Geometry: final body of the model. Coordinates: model frame, mm. Coordinates: 2 decimals unless noted, no trailing zeros. Use a Markdown table: item, result. Add a question column.
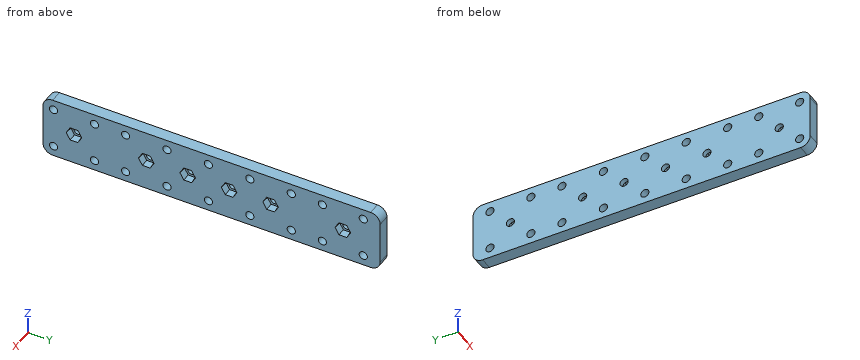
```python
from build123d import *

# Parameters (mm, degrees)
ESQUISSE2_R             = 1.7
BOSS_EXTRU_1_DEPTH      = 5
ENL_V_MAT_EXTRU_1_DEPTH = 3
ENL_V_MAT_EXTRU_1_TAPER = 5


with BuildPart() as part:
    # Esquisse2 → Boss.-Extru.1 (new body)
    with BuildSketch(Plane(origin=(0, 0, 0), x_dir=(0, 0, -1), z_dir=(1, 0, 0))):
        with BuildLine():
            Line((-25.6, -133.893899255), (-25.6, -1.893899255))
            ThreePointArc((-25.6, -1.893899255), (-24.428427125, 0.93452787), (-21.6, 2.106100745))
            Line((-21.6, 2.106100745), (-4.004577751, 2.106100745))
            ThreePointArc((-4.004577751, 2.106100745), (-1.176198229, 0.934575472), (-0.004577753, -1.893764615))
            Line((-0.004577753, -1.893764615), (-0.000134644, -133.893764615))
            ThreePointArc((-0.000134644, -133.893764615), (-1.171659915, -136.722278777), (-4.000134642, -137.893899255))
            Line((-4.000134642, -137.893899255), (-21.6, -137.893899255))
            ThreePointArc((-21.6, -137.893899255), (-24.428427125, -136.72232638), (-25.6, -133.893899255))
        make_face()
        with Locations((-21.285281374, -103.629375049)):
            Circle(ESQUISSE2_R, mode=Mode.SUBTRACT)
        with Locations((-4.314718626, -103.629375049)):
            Circle(ESQUISSE2_R, mode=Mode.SUBTRACT)
        with Locations((-4.314718626, -86.427328272)):
            Circle(ESQUISSE2_R, mode=Mode.SUBTRACT)
        with Locations((-21.285281374, -86.427328272)):
            Circle(ESQUISSE2_R, mode=Mode.SUBTRACT)
        with Locations((-21.285281374, -133.513633034)):
            Circle(ESQUISSE2_R, mode=Mode.SUBTRACT)
        with Locations((-4.314718626, -133.513633034)):
            Circle(ESQUISSE2_R, mode=Mode.SUBTRACT)
        with Locations((-4.314718626, -69.225281495)):
            Circle(ESQUISSE2_R, mode=Mode.SUBTRACT)
        with Locations((-21.285281374, -69.225281495)):
            Circle(ESQUISSE2_R, mode=Mode.SUBTRACT)
        with Locations((-4.314718626, -52.023234718)):
            Circle(ESQUISSE2_R, mode=Mode.SUBTRACT)
        with Locations((-21.285281374, -52.023234718)):
            Circle(ESQUISSE2_R, mode=Mode.SUBTRACT)
        with Locations((-4.314718626, -34.821187941)):
            Circle(ESQUISSE2_R, mode=Mode.SUBTRACT)
        with Locations((-21.285281374, -34.821187941)):
            Circle(ESQUISSE2_R, mode=Mode.SUBTRACT)
        with Locations((-21.285281374, -4.936929955)):
            Circle(ESQUISSE2_R, mode=Mode.SUBTRACT)
        with Locations((-4.314718626, -4.936929955)):
            Circle(ESQUISSE2_R, mode=Mode.SUBTRACT)
        with Locations((-4.314718626, -116.543070286)):
            Circle(ESQUISSE2_R, mode=Mode.SUBTRACT)
        with Locations((-21.285281374, -116.543070286)):
            Circle(ESQUISSE2_R, mode=Mode.SUBTRACT)
        with Locations((-4.314718626, -21.907492704)):
            Circle(ESQUISSE2_R, mode=Mode.SUBTRACT)
        with Locations((-21.285281374, -21.907492704)):
            Circle(ESQUISSE2_R, mode=Mode.SUBTRACT)
        with Locations((-12.8, -13.422211329)):
            Circle(ESQUISSE2_R, mode=Mode.SUBTRACT)
        with Locations((-12.8, -43.422211329)):
            Circle(ESQUISSE2_R, mode=Mode.SUBTRACT)
        with Locations((-12.8, -60.624258106)):
            Circle(ESQUISSE2_R, mode=Mode.SUBTRACT)
        with Locations((-12.8, -77.826304883)):
            Circle(ESQUISSE2_R, mode=Mode.SUBTRACT)
        with Locations((-12.8, -95.02835166)):
            Circle(ESQUISSE2_R, mode=Mode.SUBTRACT)
        with Locations((-12.8, -125.02835166)):
            Circle(ESQUISSE2_R, mode=Mode.SUBTRACT)
    extrude(amount=BOSS_EXTRU_1_DEPTH)

    # Esquisse3 → Enlèv. mat.-Extru.1 (cut)
    with BuildSketch(Plane(origin=(5, 0, 0), x_dir=(0, 0, -1), z_dir=(1, 0, 0))):
        Polygon((-12.8, -10.189049822), (-15.6, -11.805630576), (-15.6, -15.038792083), (-12.8, -16.655372837), (-10, -15.038792083), (-10, -11.805630576), align=None)
        Polygon((-12.8, -40.189049822), (-15.6, -41.805630576), (-15.6, -45.038792083), (-12.8, -46.655372837), (-10, -45.038792083), (-10, -41.805630576), align=None)
        Polygon((-12.8, -57.391096599), (-15.6, -59.007677352), (-15.6, -62.24083886), (-12.8, -63.857419614), (-10, -62.24083886), (-10, -59.007677352), align=None)
        Polygon((-12.8, -74.593143376), (-15.6, -76.209724129), (-15.6, -79.442885637), (-12.8, -81.059466391), (-10, -79.442885637), (-10, -76.209724129), align=None)
        Polygon((-12.8, -91.795190153), (-15.6, -93.411770906), (-15.6, -96.644932414), (-12.8, -98.261513168), (-10, -96.644932414), (-10, -93.411770906), align=None)
        Polygon((-12.8, -121.795190153), (-15.6, -123.411770906), (-15.6, -126.644932414), (-12.8, -128.261513168), (-10, -126.644932414), (-10, -123.411770906), align=None)
    extrude(amount=-ENL_V_MAT_EXTRU_1_DEPTH, taper=ENL_V_MAT_EXTRU_1_TAPER, mode=Mode.SUBTRACT)


solid = part.part
```
1) Section A-A (x = 1.2). Give the number of separate pieces and of enclosed holes in the cut face, then the cut area to 3 significant figures.
2) Ray query, line 1 along Z through (x, y) = (0.25, -38.5); line 2 along Z through (x, y) = (4.15, -85.5); line 3 along Z through (x, y) = (0.4, -6). Return the intervals inside material, ascending.
3) Pin query (flat end, axial travel): pin 1 (2.5 mm diameter, centred on y = -94.5, z = 13, fed in from +X). Return the tip coordinate at first contact, or that it passes through.
Values follow:
| question | item | result |
|---|---|---|
| 1 | separate pieces | 1 |
| 1 | enclosed holes | 24 |
| 1 | area | 3,350 mm² |
| 2 | line 1 | z = 0 to 25.6 |
| 2 | line 2 | z = 0 to 2.89, 5.74 to 19.86, 22.71 to 25.6 |
| 2 | line 3 | z = 0 to 2.99, 5.64 to 19.96, 22.61 to 25.6 |
| 3 | pin 1 | stops at x = 2 |
